Design review of the part built by this model. Coordinates are the model's own, in mm. A direction names the side the tool comes from. Coordinates: 2 decimals unless noted, no trailing zeros. Write each loop counter-clockwise with the first axis right and the second up, starting at its lowest first coordinate (ties: lowest second). Pieces come first, ordered by that corner, then holes. Notation, with made-up numbers: (-25.5, -3) - (-3.5, -3) arc R17 cw to (-3.5, 5) - close; hole circle Ø3 at (45, 71.25). An arc over 180 degrees is marked (long way). One line per item, written item: value.
from build123d import *

# Parameters (mm, degrees)
F0_W     = 1524
F0_H     = 152.4
F1_DEPTH = 25.4
F2_W     = 25.4
F2_H     = 215.900069
F3_DEPTH = 6.35
F4_R     = 3.175
F5_DEPTH = 25.4


with BuildPart() as f1:
    # F0 (on Top) → F1 (new body)
    with BuildSketch(Plane.XY):
        with Locations((762, 76.2)):
            Rectangle(F0_W, F0_H)
    extrude(amount=F1_DEPTH)

    # F2 (on Top) → F3 (cut)
    with BuildSketch(Plane.XY):
        with Locations((38.1, 77.015946)):
            Rectangle(F2_W, F2_H)
        with Locations((520.7, 77.015946)):
            Rectangle(F2_W, F2_H)
        with Locations((1003.3, 77.015946)):
            Rectangle(F2_W, F2_H)
        with Locations((1485.9, 77.015946)):
            Rectangle(F2_W, F2_H)
    extrude(amount=F3_DEPTH, mode=Mode.SUBTRACT)

    # F4 (on Front) → F5 (cut)
    with BuildSketch(Plane.XZ):
        with Locations((101.6, 12.7)):
            Circle(F4_R)
        with Locations((406.4, 12.7)):
            Circle(F4_R)
        with Locations((762, 12.7)):
            Circle(F4_R)
        with Locations((1117.6, 12.7)):
            Circle(F4_R)
        with Locations((1422.4, 12.7)):
            Circle(F4_R)
    extrude(amount=-F5_DEPTH, mode=Mode.SUBTRACT)


solid = f1.part
1. Insertion check: pin 1 Ø1.9 at (y, z) = (108, 2) entering from -X; pin 2 Ø5.5 at (x, z) = (1422.4, 12.7) entering from -Y; pin 3 Ø7.5 at (x, y) = (1486.5, 77.5) entering from -Z. Each pin has a flat end and moves straight along its axis. Give the tip position at first contact, or say it passes through.
Answer block:
pin 1: stops at x = 0
pin 2: stops at y = 25.4
pin 3: stops at z = 6.35
2. Wall thickness on line 1 along X through (y, z) = (17.5, 1); line 2 along Z through (x, y) = (101, 17); line 3 along Z through (x, y) = (101.6, 8.25) (3 decimals): over which ranges is each line inside the solid? List them lowest first.
Answer block:
line 1: x = 0 to 25.4, 50.8 to 508, 533.4 to 990.6, 1016 to 1473.2, 1498.6 to 1524
line 2: z = 0 to 9.58, 15.82 to 25.4
line 3: z = 0 to 9.525, 15.875 to 25.4
3. For faces 1 (the face through (1003, 77, 6.35)), 2 (the face through (276, 77, 0)), list the 3-axis set-ups (+Z, -Z, +X, -X, +Y, -Y) from which the entire face can be reached by the end or side of a thin tool; tool diameter is ignored.
Answer block:
face 1: -Z, +Y, -Y
face 2: -Z, +X, -X, +Y, -Y
4. Consider section A-A, the plane y = 114. Write out the cut boundary in (x, z).
Answer block:
outline: (0, 0) - (25.4, 0) - (25.4, 6.35) - (50.8, 6.35) - (50.8, 0) - (508, 0) - (508, 6.35) - (533.4, 6.35) - (533.4, 0) - (990.6, 0) - (990.6, 6.35) - (1016, 6.35) - (1016, 0) - (1473.2, 0) - (1473.2, 6.35) - (1498.6, 6.35) - (1498.6, 0) - (1524, 0) - (1524, 25.4) - (0, 25.4) - close
